from build123d import *

# Parameters (mm, degrees)
SKETCH1_R               = 1.5
SKETCH1_R_2             = 3.95
MAIN_BODY_LINK_B1_DEPTH = 3
CUT_EXTRUDE1_REACH      = 168.945
PULLEYIDLER_DEPTH       = 3
FILLET1_R               = 1


with BuildPart() as part:
    # Sketch1 → Main Body Link B1 (new body)
    with BuildSketch(Plane.XY):
        with BuildLine():
            Line((0, 83.474052381), (9.1, 83.474052381))
            Line((9.1, 83.474052381), (9.1, 89.474052381))
            Line((9.1, 89.474052381), (11.1, 89.474052381))
            Line((11.1, 89.474052381), (11.1, 83.474052381))
            Line((11.1, 83.474052381), (20.2, 83.474052381))
            Line((20.2, 83.474052381), (20.2, 90.874052381))
            Line((20.2, 90.874052381), (17.986683974, 148.383116621))
            ThreePointArc((17.986683974, 148.383116621), (0, 165.690874165), (-17.986683974, 148.383116621))
            Line((-17.986683974, 148.383116621), (-20.2, 90.874052381))
            Line((-20.2, 90.874052381), (-20.2, 83.474052381))
            Line((-20.2, 83.474052381), (-11.1, 83.474052381))
            Line((-11.1, 83.474052381), (-11.1, 89.474052381))
            Line((-11.1, 89.474052381), (-9.1, 89.474052381))
            Line((-9.1, 89.474052381), (-9.1, 83.474052381))
            Line((-9.1, 83.474052381), (0, 83.474052381))
        make_face()
        with Locations((5.2, 88.124052381)):
            Circle(SKETCH1_R, mode=Mode.SUBTRACT)
        with Locations((15, 88.124052381)):
            Circle(SKETCH1_R, mode=Mode.SUBTRACT)
        with Locations((-15, 88.124052381)):
            Circle(SKETCH1_R, mode=Mode.SUBTRACT)
        with Locations((-5.2, 88.124052381)):
            Circle(SKETCH1_R, mode=Mode.SUBTRACT)
        with Locations((0, 147.690874165)):
            Circle(SKETCH1_R_2, mode=Mode.SUBTRACT)
    extrude(amount=MAIN_BODY_LINK_B1_DEPTH)

    # Sketch2 → Cut-Extrude1 (cut, up to next)
    with BuildSketch(Plane.XY.offset(3), mode=Mode.PRIVATE) as cut_extrude1_sk1:
        Polygon((-3.278172542, 117.482670232), (12, 128.172168466), (12, 106.793171999), align=None)
    cut_extrude1_tool1 = extrude(cut_extrude1_sk1.sketch, amount=-CUT_EXTRUDE1_REACH, mode=Mode.PRIVATE) & part.part
    # Sketch2 → Cut-Extrude1 (cut, up to next)
    with BuildSketch(Plane.XY.offset(3), mode=Mode.PRIVATE) as cut_extrude1_sk2:
        with BuildLine():
            ThreePointArc((-12, 134.2744663), (-7.774454217, 131.456408925), (-2.929911079, 129.930929878))
            Line((-2.929911079, 129.930929878), (-12, 123.584968066))
            Line((-12, 123.584968066), (-12, 134.2744663))
        make_face()
    cut_extrude1_tool2 = extrude(cut_extrude1_sk2.sketch, amount=-CUT_EXTRUDE1_REACH, mode=Mode.PRIVATE) & part.part
    # Sketch2 → Cut-Extrude1 (cut, up to next)
    with BuildSketch(Plane.XY.offset(3), mode=Mode.PRIVATE) as cut_extrude1_sk3:
        Polygon((-12, 111.380372399), (-12, 100.690874165), (3.278172542, 100.690874165), align=None)
    cut_extrude1_tool3 = extrude(cut_extrude1_sk3.sketch, amount=-CUT_EXTRUDE1_REACH, mode=Mode.PRIVATE) & part.part
    add(cut_extrude1_tool1.solids().sort_by_distance((6.907276, 117.48267, 3))[0], mode=Mode.SUBTRACT)
    add(cut_extrude1_tool2.solids().sort_by_distance((-9.12997, 128.978342, 3))[0], mode=Mode.SUBTRACT)
    add(cut_extrude1_tool3.solids().sort_by_distance((-6.907276, 104.25404, 3))[0], mode=Mode.SUBTRACT)

    # Sketch3 → PulleyIdler (cut)
    with BuildSketch(Plane.XY.offset(3)):
        with BuildLine():
            Line((-4.812543936, 110.623218529), (7.477908291, 102.024103222))
            ThreePointArc((7.477908291, 102.024103222), (9.566865044, 102.393236914), (9.197731352, 104.482193668))
            Line((9.197731352, 104.482193668), (-3.092720875, 113.081308975))
            ThreePointArc((-3.092720875, 113.081308975), (-5.181677628, 112.712175283), (-4.812543936, 110.623218529))
        make_face()
    extrude(amount=-PULLEYIDLER_DEPTH, mode=Mode.SUBTRACT)

    # Fillet1
    fillet1_edges = [part.edges().sort_by_distance(p)[0] for p in [
        (-3.278172542, 117.482670232, 1.5),
        (12, 128.172168466, 1.5),
        (12, 106.793171999, 1.5),
        (-12, 134.2744663, 1.5),
        (-2.929911079, 129.930929878, 1.5),
        (-12, 123.584968066, 1.5),
        (-12, 111.380372399, 1.5),
        (3.278172542, 100.690874165, 1.5),
        (-12, 100.690874165, 1.5),
    ]]
    fillet(fillet1_edges, radius=FILLET1_R)


solid = part.part
Model file for the job. Use its own axes, mm. A direction names the side the tool comes from. Coordinates: 2 decimals unless noted, no trailing zeros. Loops run counter-clockwise (first coordinate to the right, second up) from the corner with the lowest first, then second, coordinate; pieces in that order, holes last. Notation, with made-up numbers: (-7, 26) -> (12, 26) arc R16 cw to (12, 31) -> close; hole circle Ø5 at (89, 17). An arc over 180 degrees is marked (long way). Use one line per item in the form item = value. Start each with the question number.
(1) Cut at B-B on x = 15. Give the cut face in (y, z).
(2) Tool access for faces 4 (the flat face through (10, 89.474, 1)), 5 (the flat face through (12, 118, 2)), 6 (the flat face through (-20.2, 87, 1)): list every direction of +Z, -Z, +X, -X, +Y, -Y with a clear straight run to the whole face (end or side of a thin tool).
(3) Pull direction X, two halves, no side cores. Call faces 1 (the flat face through (-19.078, 120.031, 1.479)), 2 (the cylindrical face through (-7.89, 131.512, 1.521)), 3 (the flat face through (0, 125, 3)): pulls with the +X half, pulls with the -X half, needs draft (parallel to the pull), parting line crosses it, or undercut.
(4) Cut at D-D on y = 140. Give the cut face in (x, z), and give its area (3 significant figures).
(5) Cut at A-A on x = 5.2. Give the cut face in (y, z).
(6) Probe probe 1 along Y at (x, z) = (5.5, 0.55); probe 2 along Y at (x, z) = (4, 1.9); probe 3 along Y at (x, z) = (-9, 0.4). List the from-to ranges inside material, lowest first. Write a range as from..to.
(7) Flat gauge pins, fed straight in: pin 1 (1 mm diameter, centred on y = 124, z = 2.5, fed in from +X); pin 2 (0.6 mm diameter, centred on x = -10, z = 1, fed in from -Y). Where does each tip first touch, or does it go through?
(8) Cut at C-C on z = 1.6. Give the number of separate pieces and of enclosed holes in the cut face, and give its area (3 significant figures).
Values:
q1.outline = (83.47, 0) -> (86.62, 0) -> (86.62, 3) -> (83.47, 3) -> close; (89.62, 0) -> (157.64, 0) -> (157.64, 3) -> (89.62, 3) -> close
q2.face_4 = +Z, -Z, -Y
q2.face_5 = +Z, -Z
q2.face_6 = +Z, -Z, -X, +Y, -Y
q3.face_1 = pulls with the -X half
q3.face_2 = undercut
q3.face_3 = needs draft
q4.outline = (-18.31, 0) -> (18.31, 0) -> (18.31, 3) -> (-18.31, 3) -> close
q4.area = 110 mm2
q5.outline = (83.47, 0) -> (86.62, 0) -> (86.62, 3) -> (83.47, 3) -> close; (89.62, 0) -> (103.62, 0) -> (103.62, 3) -> (89.62, 3) -> close; (107.28, 0) -> (111.55, 0) -> (111.55, 3) -> (107.28, 3) -> close; (123.41, 0) -> (164.92, 0) -> (164.92, 3) -> (123.41, 3) -> close
q6.probe_1 = 83.47..86.65, 89.59..103.41, 107.07..111.34, 123.62..164.83
q6.probe_2 = 83.47..87.22, 89.02..104.46, 108.12..112.39, 122.57..165.24
q6.probe_3 = 83.47..100.69, 109.28..125.68, 132.1..163.28
q7.pin_1 = 18.94
q7.pin_2 = 89.47
q8.separate_pieces = 1
q8.enclosed_holes = 9
q8.area = 2,540 mm2
